Read the model definition and answer for the solid it produces. Units are mm, in the model's axes. A direction names the side the tool comes from. Coordinates: 2 decimals unless noted, no trailing zeros. Write each loop counter-clockwise with the first axis right and the second up, starting at its lowest first coordinate (ties: lowest second). Pieces come first, ordered by that corner, then holes.
(1) The part is cut by section C-C, the plane z = -40. Determine the outline of the cut face in (x, y).
(2) Which of the six approach directions +Z, -Z, +X, -X, +Y, -Y give full straight-line access (tool end or side, diameter ignored) to faces 4 (the cylindrical face through (39.54, 2.96, -38.04)), 5 (the flat face through (6, 44, -11)), 6 (the flat face through (0, 26, -16)), 7 (the flat face through (5, 33, -22)), 8 (the flat face through (60, 6, -24))?
(3) Straight lines are drawn through the part: line 1 along Y through (x, z) = (1, -11); line 2 along X through (y, z) = (29, -9); line 3 along X through (y, z) = (4.2, -7.5). For each, find the intervals that lie inside material, in ascending order.
(4) The part is cut by section D-D, the plane x = 29. Determine the outline of the cut face in (y, z), and give its area (3 significant figures).
(5) The part is cut by section B-B, the plane y = 64. Determine the outline of the cut face in (x, z).
(6) Given pin 1 (1 mm diameter, centred on x = 126, z = -11.5, fed in from +Y); pin 2 (17 mm diameter, centred on x = 142.5, y = 37.5, fed in from -Z), each flat-ended and moving along its own axis, determine where each tip first touches the part or whether it passes through.
(7) Determine the mould class of faces 1 (the flat face through (76, 4, 0)), 2 (the flat face through (90.726, 2.958, -41.266)), 3 (the flat face through (147.589, 44, -11)) for opening direction X: pulls with the +X half, pulls with the -X half, needs draft (parallel to the pull), parting line crosses it, or undercut.
(8) The part is cut by section A-A, the plane y = 34. Determine the outline of the cut face in (x, z).
```python
from build123d import *

# Parameters (mm, degrees)
SKETCH1_R                       = 2.5
BOSS_EXTRUDE1_DEPTH             = 6
SKETCH2_W                       = 6
SKETCH2_H                       = 22
BOSS_EXTRUDE2_DEPTH             = 62.5
BOSS_EXTRUDE3_REACH             = 176.194
SKETCH4_W                       = 6
SKETCH4_H                       = 22
BOSS_EXTRUDE3_DIRECTION_2_REACH = 176.194
SKETCH3_R                       = 2.5
CUT_EXTRUDE2_DEPTH              = 179.555261525
BOSS_EXTRUDE4_DEPTH             = 22


with BuildPart() as part:
    # Sketch1 → Boss-Extrude1 (new body)
    with BuildSketch(Plane(origin=(0, 0, 0), x_dir=(1, 0, 0), z_dir=(0, 1, 0))):
        Polygon((32, 60), (151.12, 22), (151.12, 0), (0, 0), (0, 60), align=None)
        with Locations(Location((40.5, 40.35, 0), (0, 0, 270))):
            Circle(SKETCH1_R, mode=Mode.SUBTRACT)
        with Locations(Location((89, 7.5, 0), (0, 0, 270))):
            Circle(SKETCH1_R, mode=Mode.SUBTRACT)
    extrude(amount=BOSS_EXTRUDE1_DEPTH)

    # Sketch2 → Boss-Extrude2 (add)
    with BuildSketch(Plane(origin=(0, 6, 0), x_dir=(1, 0, 0), z_dir=(0, 1, 0))):
        with Locations((3, 11)):
            Rectangle(SKETCH2_W, SKETCH2_H)
    extrude(amount=BOSS_EXTRUDE2_DEPTH)

    # Boss-Extrude3: up to this face of the body (flat: up to its plane)
    boss_extrude3_end = Plane(part.part.faces().sort_by_distance((3, 68.5, -11))[0])
    # Sketch4 → Boss-Extrude3 (add, up to the picked face)
    with BuildSketch(Plane(origin=(0, 6, 0), x_dir=(1, 0, 0), z_dir=(0, 1, 0)), mode=Mode.PRIVATE) as boss_extrude3_sk1:
        with Locations((150.589489934, 11)):
            Rectangle(SKETCH4_W, SKETCH4_H)
    boss_extrude3_tool1 = split(extrude(boss_extrude3_sk1.sketch, amount=BOSS_EXTRUDE3_REACH, mode=Mode.PRIVATE), bisect_by=boss_extrude3_end, keep=Keep.BOTH, mode=Mode.PRIVATE)
    add(boss_extrude3_tool1.solids().sort_by(Axis((150.58949, 6, -11), (0, 1, 0)))[0])

    # Boss-Extrude3 direction 2: up to this face of the body (flat: up to its plane)
    boss_extrude3_direction_2_end = Plane(part.part.faces().sort_by_distance((63.627139695, 0, -24.235973562))[0])
    # Sketch4 → Boss-Extrude3 direction 2 (add, up to the picked face)
    with BuildSketch(Plane(origin=(0, 6, 0), x_dir=(1, 0, 0), z_dir=(0, 1, 0)), mode=Mode.PRIVATE) as boss_extrude3_direction_2_sk1:
        with Locations((150.589489934, 11)):
            Rectangle(SKETCH4_W, SKETCH4_H)
    boss_extrude3_direction_2_tool1 = split(extrude(boss_extrude3_direction_2_sk1.sketch, amount=-BOSS_EXTRUDE3_DIRECTION_2_REACH, mode=Mode.PRIVATE), bisect_by=boss_extrude3_direction_2_end, keep=Keep.BOTH, mode=Mode.PRIVATE)
    add(boss_extrude3_direction_2_tool1.solids().sort_by(Axis((150.58949, 6, -11), (0, -1, 0)))[0])

    # Sketch3 → Cut-Extrude2 (cut, through all)
    with BuildSketch(Plane.ZY):
        with Locations((-11, 64)):
            Circle(SKETCH3_R)
        with Locations((-11, 50)):
            Circle(SKETCH3_R)
    extrude(amount=-CUT_EXTRUDE2_DEPTH, mode=Mode.SUBTRACT)

    # Sketch5 → Boss-Extrude4 (add)
    with BuildSketch(Plane.XY):
        with BuildLine():
            Line((6, 21), (6, 6))
            Line((6, 6), (21, 6))
            add(Edge.make_bspline(
                [(6, 21), (8.5, 8.5), (21, 6)],
                knots=[0, 0, 0, 1, 1, 1], degree=2))
        make_face()
        with BuildLine():
            Line((132.589489934, 6), (147.589489934, 6))
            Line((147.589489934, 6), (147.589489934, 21))
            add(Edge.make_bspline(
                [(147.589489934, 21), (145.089489934, 8.5), (132.589489934, 6)],
                knots=[0, 0, 0, 1, 1, 1], degree=2))
        make_face()
    extrude(amount=-BOSS_EXTRUDE4_DEPTH)


solid = part.part
```
Computed:
1. outline: (0, 0) - (38.02, 0) - (38.02, 6) - (0, 6) - close; (42.98, 0) - (94.69, 0) - (94.69, 6) - (42.98, 6) - close
2. face 4: +Y, -Y
2. face 5: +Z, -Z, +Y
2. face 6: +Z, -Z, -X, +Y, -Y
2. face 7: -Z, +X, -X, +Y
2. face 8: -Z, +Y
3. line 1: y = 0 to 47.5, 52.5 to 61.5, 66.5 to 68.5
3. line 2: x = 0 to 6, 147.59 to 153.59
3. line 3: x = 0 to 86.5, 91.5 to 153.59
4. outline: (0, -60) - (6, -60) - (6, 0) - (0, 0) - close
4. area: 360 mm2
5. outline: (0, -22) - (6, -22) - (6, -13.5) - (0, -13.5) - close; (0, -8.5) - (6, -8.5) - (6, 0) - (0, 0) - close; (147.59, -22) - (153.59, -22) - (153.59, -13.5) - (147.59, -13.5) - close; (147.59, -8.5) - (153.59, -8.5) - (153.59, 0) - (147.59, 0) - close
6. pin 1: stops at y = 6
6. pin 2: stops at z = -22
7. face 1: needs draft
7. face 2: pulls with the +X half
7. face 3: undercut
8. outline: (0, -22) - (6, -22) - (6, 0) - (0, 0) - close; (147.59, -22) - (153.59, -22) - (153.59, 0) - (147.59, 0) - close
